from build123d import *

# Parameters (mm, degrees)
SKETCH1_R           = 5
BOSS_EXTRUDE1_DEPTH = 10
SKETCH3_W           = 10
SKETCH3_H           = 10
BOSS_EXTRUDE2_DEPTH = 7.5
SKETCH2_R           = 2
CUT_EXTRUDE1_DEPTH  = 11


with BuildPart() as part:
    # Sketch1 → Boss-Extrude1 (new body)
    with BuildSketch(Plane.XY):
        Circle(SKETCH1_R)
    extrude(amount=BOSS_EXTRUDE1_DEPTH)

    # Sketch3 → Boss-Extrude2 (add)
    with BuildSketch(Plane.XY.offset(10)):
        Rectangle(SKETCH3_W, SKETCH3_H)
    extrude(amount=-BOSS_EXTRUDE2_DEPTH)

    # Sketch2 → Cut-Extrude1 (cut, through all)
    with BuildSketch(Plane(origin=(5, 0, 0), x_dir=(0, 0, -1), z_dir=(1, 0, 0))):
        with Locations((-5, 0)):
            Circle(SKETCH2_R)
    extrude(amount=-CUT_EXTRUDE1_DEPTH, mode=Mode.SUBTRACT)


solid = part.part
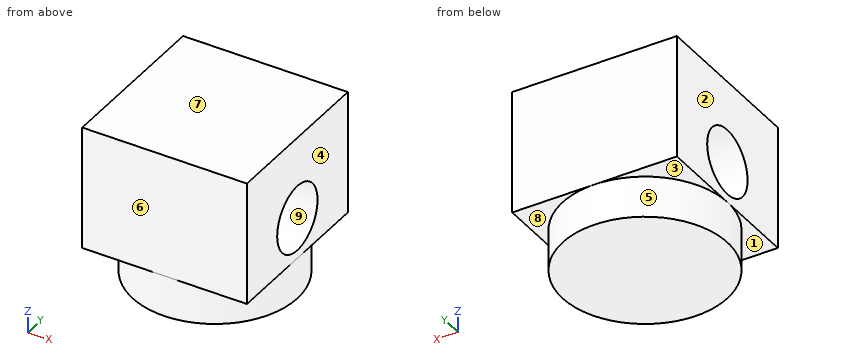
Could you check a few things on this model? Use its own coordinates, in mm. Face numbers are marked on the shaded views. A direction names the side the tool comes from. Give positions to 0.01 mm unless a question says otherwise; leave off trailing zeros. Order: outer loops, then holes, each group sorted by start corner. A loop starts at its lowest first (then second) coordinate and runs counter-clockwise, first axis right, second up.
Item 1: For the marked faces 1, 2, 3, 4 and 5, which set-ups out of +Z, -Z, +X, -X, +Y, -Y let a thin tool reach every point of the face, with its end or its side?
Item 2: If we mould it in two halves opening along Z, with no side actions, what happens to the marked faces 6, 7, 8 and 9? For each: pulls with the +Z half, pulls with the -Z half, needs draft (parallel to the pull), parting line crosses it, or undercut.
Item 3: If we section it at B-B, the plane x = 4: Write out the boundary of the cut face in (y, z).
Item 4: If we section it at A-A, the plane z = 5: Write out the boundary of the cut face in (x, y).
Item 5: I need wall thicknesses on line 1 (Y direction, x = -2.5, z = 5); line 2 (Z direction, x = 4, y = -0.25); line 3 (Z direction, x = 4, y = -1.5). Which ranges of each line are inside material? Lowest first, please.
Item 6: I'm going to push a flat-ended pin straight in: pin 1 (1.5 mm diameter, centred on x = 2.5, z = 1.5, fed in from +Y). Where does the tip first touch, or does it pass through?
Item 7: If we section it at C-C, the plane y = -3: Write out the boundary of the cut face in (x, z), plus the area to 3 significant figures.
Values:
1. face 1: -Z, -X, -Y
1. face 2: +Z, -Z, -X, +Y, -Y
1. face 3: -Z, -X, +Y
1. face 4: +Z, -Z, +X, +Y, -Y
1. face 5: -Z
2. face 6: needs draft
2. face 7: pulls with the +Z half
2. face 8: pulls with the -Z half
2. face 9: undercut
3. outline: (-5, 2.5) - (-3, 2.5) - (-3, 0) - (3, 0) - (3, 2.5) - (5, 2.5) - (5, 10) - (-5, 10) - close; hole circle Ø4 at (0, 5)
4. outline: (-5, -5) - (5, -5) - (5, -2) - (-5, -2) - close; (-5, 2) - (5, 2) - (5, 5) - (-5, 5) - close
5. line 1: y = -5 to -2, 2 to 5
5. line 2: z = 0 to 3.02, 6.98 to 10
5. line 3: z = 0 to 3.68, 6.32 to 10
6. pin 1: stops at y = 4.68
7. outline: (-5, 2.5) - (-4, 2.5) - (-4, 0) - (4, 0) - (4, 2.5) - (5, 2.5) - (5, 10) - (-5, 10) - close
7. area: 95.0 mm2
